Source: CAD feature listing. Evaluate the final solid. Frame: model axes, mm. A direction names the side the tool comes from. Round coordinates to 2 decimals unless told otherwise and drop trailing zeros. Order: outer loops, then holes, each group sorted by start corner. A loop starts at its lowest first (then second) coordinate and runs counter-clockwise, first axis right, second up. Notation, with made-up numbers: (78, 1) -> (124, 1) arc R23 cw to (124, 35) -> close; hole circle Ø11 at (58.25, 12.5). An arc over 180 degrees is marked (long way). Use a Markdown table: item, result. Add a question column.
```python
from build123d import *

# Parameters (mm, degrees)
EXTRUDE_1_DEPTH     = 30
CUT_EXTRUDE_3_REACH = 40
SKETCH_4_R          = 2.75
SKETCH_4_R_2        = 3.25
CUT_EXTRUDE_4_REACH = 5
SKETCH_5_R          = 3.25


with BuildPart() as part:
    # 草图1 → 凸台-拉伸1 (new body)
    with BuildSketch(Plane.XY):
        Polygon((0, 0), (0, 38), (-3, 38), (-3, 3), (-38, 3), (-38, 0), align=None)
    extrude(amount=EXTRUDE_1_DEPTH)

    # 草图4 → 切除-拉伸3 (cut, up to next)
    with BuildSketch(Plane(origin=(0, 0, 0), x_dir=(0, 0, -1), z_dir=(1, 0, 0)), mode=Mode.PRIVATE) as cut_extrude_3_sk1:
        with Locations((-10, 29)):
            Circle(SKETCH_4_R)
    cut_extrude_3_tool1 = extrude(cut_extrude_3_sk1.sketch, amount=-CUT_EXTRUDE_3_REACH, mode=Mode.PRIVATE) & part.part
    add(cut_extrude_3_tool1.solids().sort_by_distance((0, 29, 10))[0], mode=Mode.SUBTRACT)
    # 草图4 → 切除-拉伸3 (cut, up to next)
    with BuildSketch(Plane(origin=(0, 0, 0), x_dir=(0, 0, -1), z_dir=(1, 0, 0)), mode=Mode.PRIVATE) as cut_extrude_3_sk2:
        with Locations((-10, 19)):
            Circle(SKETCH_4_R_2)
    cut_extrude_3_tool2 = extrude(cut_extrude_3_sk2.sketch, amount=-CUT_EXTRUDE_3_REACH, mode=Mode.PRIVATE) & part.part
    add(cut_extrude_3_tool2.solids().sort_by_distance((0, 19, 10))[0], mode=Mode.SUBTRACT)
    # 草图4 → 切除-拉伸3 (cut, up to next)
    with BuildSketch(Plane(origin=(0, 0, 0), x_dir=(0, 0, -1), z_dir=(1, 0, 0)), mode=Mode.PRIVATE) as cut_extrude_3_sk3:
        with Locations((-10, 9)):
            Circle(SKETCH_4_R)
    cut_extrude_3_tool3 = extrude(cut_extrude_3_sk3.sketch, amount=-CUT_EXTRUDE_3_REACH, mode=Mode.PRIVATE) & part.part
    add(cut_extrude_3_tool3.solids().sort_by_distance((0, 9, 10))[0], mode=Mode.SUBTRACT)
    # 草图4 → 切除-拉伸3 (cut, up to next)
    with BuildSketch(Plane(origin=(0, 0, 0), x_dir=(0, 0, -1), z_dir=(1, 0, 0)), mode=Mode.PRIVATE) as cut_extrude_3_sk4:
        with Locations((-20, 29)):
            Circle(SKETCH_4_R)
    cut_extrude_3_tool4 = extrude(cut_extrude_3_sk4.sketch, amount=-CUT_EXTRUDE_3_REACH, mode=Mode.PRIVATE) & part.part
    add(cut_extrude_3_tool4.solids().sort_by_distance((0, 29, 20))[0], mode=Mode.SUBTRACT)
    # 草图4 → 切除-拉伸3 (cut, up to next)
    with BuildSketch(Plane(origin=(0, 0, 0), x_dir=(0, 0, -1), z_dir=(1, 0, 0)), mode=Mode.PRIVATE) as cut_extrude_3_sk5:
        with Locations((-20, 9)):
            Circle(SKETCH_4_R)
    cut_extrude_3_tool5 = extrude(cut_extrude_3_sk5.sketch, amount=-CUT_EXTRUDE_3_REACH, mode=Mode.PRIVATE) & part.part
    add(cut_extrude_3_tool5.solids().sort_by_distance((0, 9, 20))[0], mode=Mode.SUBTRACT)

    # 草图5 → 切除-拉伸4 (cut, up to next)
    with BuildSketch(Plane(origin=(0, 3, 0), x_dir=(1, 0, 0), z_dir=(0, 1, 0)), mode=Mode.PRIVATE) as cut_extrude_4_sk1:
        with Locations((-20.5, -15)):
            Circle(SKETCH_5_R)
    cut_extrude_4_tool1 = extrude(cut_extrude_4_sk1.sketch, amount=-CUT_EXTRUDE_4_REACH, mode=Mode.PRIVATE) & part.part
    add(cut_extrude_4_tool1.solids().sort_by_distance((-20.5, 3, 15))[0], mode=Mode.SUBTRACT)


solid = part.part
```
1) Section C-C on y = 18. Output: boundary loops of the cut face in (x, z), then the cut area to 3 significant figures.
2) Line query: probe 1 along Y at (x, z) = (-1.8, 10); probe 2 along Y at (x, z) = (-1.25, 20); probe 3 along Z at (x, y) = (-20.5, 2.2). Output: solid intervals per line, ascending. Write a range as from..to.
3) First-contact query: pin 1 Ø8 at (y, z) = (20.5, 20) entering from -X; pin 2 Ø10.5 at (x, z) = (-20.5, 15) entering from +Y. Flat tips, straight axial feed; report the tip coordinate or a pass-through.
4) Draft query along Y for faces 1 (the cylindrical face through (-1.479, 9.121, 22.747)), 2 (the flat face through (-20, 3, 11)), 3 (the cylindrical face through (-1.479, 31.727, 10.358)), 4 (the cylindrical face through (-22.895, 1.521, 12.803)). Return one class per face: pulls with the +Y half, pulls with the -Y half, needs draft (parallel to the pull), parting line crosses it, or undercut.
5) Section D-D on z = 20. Output: boundary loops of the cut face in (x, y), then the cut area to 3 significant figures.
6) Section B-B on z = 10. Output: boundary loops of the cut face in (x, y).
7) Reachability of faces 5 (the cylindrical face through (-1.479, 29.121, 22.747)), 6 (the flat face through (-3, 21, 15)) from +Z, -Z, +X, -X, +Y, -Y: full face, straight path, thin tool, end or side. Return the list, or none.
8) Section A-A on x = -20.5. Output: boundary loops of the cut face in (y, z).
Conclusion:
| question | item | result |
|---|---|---|
| 1 | outline | (-3, 0) -> (0, 0) -> (0, 6.91) -> (-3, 6.91) -> close; (-3, 13.09) -> (0, 13.09) -> (0, 30) -> (-3, 30) -> close |
| 1 | area | 71.4 mm^2 |
| 2 | probe 1 | y = 0..6.25, 11.75..15.75, 22.25..26.25, 31.75..38 |
| 2 | probe 2 | y = 0..6.25, 11.75..26.25, 31.75..38 |
| 2 | probe 3 | z = 0..11.75, 18.25..30 |
| 3 | pin 1 | stops at x = -3 |
| 3 | pin 2 | stops at y = 3 |
| 4 | face 1 | undercut |
| 4 | face 2 | pulls with the +Y half |
| 4 | face 3 | undercut |
| 4 | face 4 | needs draft |
| 5 | outline | (-38, 0) -> (0, 0) -> (0, 6.25) -> (-3, 6.25) -> (-3, 3) -> (-38, 3) -> close; (-3, 11.75) -> (0, 11.75) -> (0, 26.25) -> (-3, 26.25) -> close; (-3, 31.75) -> (0, 31.75) -> (0, 38) -> (-3, 38) -> close |
| 5 | area | 186 mm^2 |
| 6 | outline | (-38, 0) -> (0, 0) -> (0, 6.25) -> (-3, 6.25) -> (-3, 3) -> (-38, 3) -> close; (-3, 11.75) -> (0, 11.75) -> (0, 15.75) -> (-3, 15.75) -> close; (-3, 22.25) -> (0, 22.25) -> (0, 26.25) -> (-3, 26.25) -> close; (-3, 31.75) -> (0, 31.75) -> (0, 38) -> (-3, 38) -> close |
| 7 | face 5 | +X, -X |
| 7 | face 6 | +Z, -Z, -X, +Y |
| 8 | outline | (0, 0) -> (3, 0) -> (3, 11.75) -> (0, 11.75) -> close; (0, 18.25) -> (3, 18.25) -> (3, 30) -> (0, 30) -> close |
